from build123d import *

# Parameters (mm, degrees)
SKETCH_1_W          = 18
SKETCH_1_H          = 29.7
EXTRUDE_1_DEPTH     = 27.7
SKETCH_2_R          = 2.075
CUT_EXTRUDE_1_DEPTH = 27.7
FILLET_1_R          = 3
SKETCH_3_R          = 4
CUT_EXTRUDE_2_DEPTH = 27.7


with BuildPart() as part:
    # 草图1 → 凸台-拉伸1 (new body)
    with BuildSketch(Plane(origin=(0, 0, 0), x_dir=(1, 0, 0), z_dir=(0, 1, 0))):
        Rectangle(SKETCH_1_W, SKETCH_1_H)
    extrude(amount=EXTRUDE_1_DEPTH)

    # 草图2 → 切除-拉伸1 (cut)
    with BuildSketch(Plane(origin=(0, 27.7, 0), x_dir=(1, 0, 0), z_dir=(0, 1, 0))):
        with Locations((5, 7.5)):
            Circle(SKETCH_2_R)
        with Locations((-5, 7.5)):
            Circle(SKETCH_2_R)
        with Locations((-5, -7.5)):
            Circle(SKETCH_2_R)
        with Locations((5, -7.5)):
            Circle(SKETCH_2_R)
    extrude(amount=-CUT_EXTRUDE_1_DEPTH, mode=Mode.SUBTRACT)

    # 圆角1
    fillet_1_edges = [part.edges().sort_by_distance(p)[0] for p in [
        (9, 13.85, 14.85),
        (-9, 13.85, 14.85),
        (-9, 13.85, -14.85),
        (9, 13.85, -14.85),
    ]]
    fillet(fillet_1_edges, radius=FILLET_1_R)

    # 草图3 → 切除-拉伸2 (cut)
    with BuildSketch(Plane(origin=(0, 27.7, 0), x_dir=(1, 0, 0), z_dir=(0, 1, 0))):
        Circle(SKETCH_3_R)
    extrude(amount=-CUT_EXTRUDE_2_DEPTH, mode=Mode.SUBTRACT)


solid = part.part
Check sheet for the modelled part. Datum: model origin and axes. Units: mm. Give positions to 0.01 mm unless a question says otherwise; leave off trailing zeros. Loops run counter-clockwise (first coordinate to the right, second up) from the corner with the lowest first, then second, coordinate; pieces in that order, holes last. Notation, with made-up numbers: M -32.75,85.25 L -18.75,85.25 A32 cw -18.75,120.25 Z; hole C -22,-3 d7. An arc over 180 degrees is marked long. Return JSON: item names as keys, results as strings. Group by question number.
1. Go/stop test with a flat-tipped pin: pin 1 (1 mm diameter, centred on x = 7, y = 4, fed in from +Z). Record where the tip stops, or that it passes through.
2. Mould release check, pull along Z, two halves, no side actions. Record for faces 1 (the flat face through (-9, 14, 0)), 2 (the cylindrical face through (8.1, 14.04, -13.99)), 3 (the cylindrical face through (4.55, 14.044, 9.526)), 4 (the cylindrical face through (-0.867, 14.044, 3.905)): released by +Z, released by -Z, zero draft, split by the parting line, or undercut.
3. Cross-section at C-C on z = 0. Record the boundary of the cut face in (x, y).
4. Cross-section at D-D on z = 7.5. Record the boundary of the cut face in (x, y) (3 decimals), plus the area to 3 significant figures.
5. Cross-section at B-B on y = 19. Record the boundary of the cut face in (x, z) (3 decimals), plus the area to 3 significant figures.
6. Thickness scan on L1, parallel to Z at x = 5, y = 13.75 (3 decimals); L2, parallel to X at y = 13.5, z = 7.5 (3 decimals); L3, parallel to Z at x = 0, y = 15. Record the ranges inside material, lowest first.
7. Cross-section at A-A on x = 0. Record the boundary of the cut face in (y, z), plus the area to 3 significant figures.
Return value:
{
 "1": {"pin 1": "z = 14.81"},
 "2": {"face 1": "zero draft", "face 2": "released by -Z", "face 3": "undercut", "face 4": "undercut"},
 "3": {"outline": "M -9,0 L -4,0 L -4,27.7 L -9,27.7 Z; M 4,0 L 9,0 L 9,27.7 L 4,27.7 Z"},
 "4": {"outline": "M -9,0 L -7.075,0 L -7.075,27.7 L -9,27.7 Z; M -2.925,0 L 2.925,0 L 2.925,27.7 L -2.925,27.7 Z; M 7.075,0 L 9,0 L 9,27.7 L 7.075,27.7 Z", "area": "269 mm^2"},
 "5": {"outline": "M -9,-11.85 A3 ccw -6,-14.85 L 6,-14.85 A3 ccw 9,-11.85 L 9,11.85 A3 ccw 6,14.85 L -6,14.85 A3 ccw -9,11.85 Z; hole C -5,-7.5 d4.15; hole C -5,7.5 d4.15; hole C 0,0 d8; hole C 5,-7.5 d4.15; hole C 5,7.5 d4.15", "area": "423 mm^2"},
 "6": {"L1": "-14.85 to -9.575, -5.425 to 5.425, 9.575 to 14.85", "L2": "-9 to -7.075, -2.925 to 2.925, 7.075 to 9", "L3": "-14.85 to -4, 4 to 14.85"},
 "7": {"outline": "M 0,-14.85 L 27.7,-14.85 L 27.7,-4 L 0,-4 Z; M 0,4 L 27.7,4 L 27.7,14.85 L 0,14.85 Z", "area": "601 mm^2"}
}
